from build123d import *

# Parameters (mm, degrees)
EXTRUDE_1_DEPTH = 1.5
FILLET_4_R      = 10
FILLET_7_R      = 1.5
FILLET_8_R      = 3
CHAMFER_1_SIZE  = 0.1
FILLET_9_R      = 2
FILLET_10_R     = 0.5


with BuildPart() as part:
    # 草图1 → 凸台-拉伸1 (new, symmetric)
    with BuildSketch(Plane.XY):
        with BuildLine():
            Line((-130, 3.05), (-130, 14.015709242))
            ThreePointArc((-130, 14.015709242), (-134.003306479, 13.533897344), (-138, 13))
            ThreePointArc((-138, 13), (-144, 12.000000001), (-150, 13))
            Line((-150, 13), (-156.350852961, 24))
            Line((-156.350852961, 24), (-182, 24))
            Line((-182, 24), (-187.773502692, 14))
            Line((-187.773502692, 14), (-189.773502692, 14))
            Line((-189.773502692, 14), (-192.082903768, 18))
            Line((-192.082903768, 18), (-213.75055535, 18))
            Line((-213.75055535, 18), (-220, 7.175644347))
            Line((-220, 7.175644347), (-220, 5.05))
            Line((-220, 5.05), (-215.5, 5.05))
            Line((-215.5, 5.05), (-215.5, 8.3))
            Line((-215.5, 8.3), (-213, 8.3))
            Line((-213, 8.3), (-210.575128869, 12.5))
            Line((-210.575128869, 12.5), (-195.258330249, 12.5))
            Line((-195.258330249, 12.5), (-192.948929172, 8.5))
            Line((-192.948929172, 8.5), (-186.581793069, 8.5))
            Line((-186.581793069, 8.5), (-184.58993464, 5.05))
            Line((-184.58993464, 5.05), (-174.637306696, 5.05))
            Line((-174.637306696, 5.05), (-177.812733177, 10.55))
            Line((-177.812733177, 10.55), (-181.41450816, 10.55))
            Line((-181.41450816, 10.55), (-182.41450816, 12.282050807))
            Line((-182.41450816, 12.282050807), (-178.824573519, 18.5))
            Line((-178.824573519, 18.5), (-159.526279442, 18.5))
            Line((-159.526279442, 18.5), (-153.637306696, 8.3))
            Line((-153.637306696, 8.3), (-150.937306696, 8.3))
            Line((-150.937306696, 8.3), (-150.937306696, 3.05))
            Line((-150.937306696, 3.05), (-150.937306696, -3.05))
            Line((-150.937306696, -3.05), (-150.937306696, -8.3))
            Line((-150.937306696, -8.3), (-153.637306696, -8.3))
            Line((-153.637306696, -8.3), (-159.526279442, -18.5))
            Line((-159.526279442, -18.5), (-178.824573519, -18.5))
            Line((-178.824573519, -18.5), (-182.41450816, -12.282050807))
            Line((-182.41450816, -12.282050807), (-181.41450816, -10.55))
            Line((-181.41450816, -10.55), (-177.812733177, -10.55))
            Line((-177.812733177, -10.55), (-174.637306696, -5.05))
            Line((-174.637306696, -5.05), (-184.58993464, -5.05))
            Line((-184.58993464, -5.05), (-186.581793069, -8.5))
            Line((-186.581793069, -8.5), (-192.948929172, -8.5))
            Line((-192.948929172, -8.5), (-195.258330249, -12.5))
            Line((-195.258330249, -12.5), (-210.575128869, -12.5))
            Line((-210.575128869, -12.5), (-213, -8.3))
            Line((-213, -8.3), (-215.5, -8.3))
            Line((-215.5, -8.3), (-215.5, -5.05))
            Line((-215.5, -5.05), (-220, -5.05))
            Line((-220, -5.05), (-220, -7.175644347))
            Line((-220, -7.175644347), (-213.75055535, -18))
            Line((-213.75055535, -18), (-192.082903768, -18))
            Line((-192.082903768, -18), (-189.773502692, -14))
            Line((-189.773502692, -14), (-187.773502692, -14))
            Line((-187.773502692, -14), (-182, -24))
            Line((-182, -24), (-156.350852961, -24))
            Line((-156.350852961, -24), (-150, -13))
            ThreePointArc((-150, -13), (-144, -12), (-138, -13))
            ThreePointArc((-138, -13), (-134.003306479, -13.533897343), (-130, -14.015709241))
            Line((-130, -14.015709242), (-130, -3.05))
            Line((-130, -3.05), (-145.937306696, -3.05))
            Line((-145.937306696, -3.05), (-145.937306696, 3.05))
            Line((-145.937306696, 3.05), (-130, 3.05))
        make_face()
    extrude(amount=EXTRUDE_1_DEPTH, both=True)

    # 圆角4
    fillet_4_edges = [part.edges().sort_by_distance(p)[0] for p in [
        (-138, 13, 0),
        (-138, -13, 0),
        (-150, -13, 0),
        (-150, 13, 0),
    ]]
    fillet(fillet_4_edges, radius=FILLET_4_R)

    # 圆角7
    fillet_7_edges = [part.edges().sort_by_distance(p)[0] for p in [
        (-187.773502692, -14, 0),
        (-189.773502692, -14, 0),
        (-210.575128869, -12.5, 0),
        (-195.258330249, -12.5, 0),
        (-186.581793069, -8.5, 0),
        (-181.41450816, -10.55, 0),
        (-182.41450816, -12.282050807, 0),
        (-178.824573519, -18.5, 0),
        (-159.526279442, -18.5, 0),
        (-159.526279442, 18.5, 0),
        (-178.824573519, 18.5, 0),
        (-182.41450816, 12.282050807, 0),
        (-181.41450816, 10.55, 0),
        (-186.581793069, 8.5, 0),
        (-195.258330249, 12.5, 0),
        (-210.575128869, 12.5, 0),
        (-189.773502692, 14, 0),
        (-187.773502692, 14, 0),
    ]]
    fillet(fillet_7_edges, radius=FILLET_7_R)

    # 圆角8
    fillet_8_edges = [part.edges().sort_by_distance(p)[0] for p in [
        (-156.350852961, -24, 0),
        (-182, -24, 0),
        (-192.082903768, -18, 0),
        (-213.75055535, -18, 0),
        (-192.948929172, -8.5, 0),
        (-184.58993464, -5.05, 0),
        (-177.812733177, -10.55, 0),
        (-177.812733177, 10.55, 0),
        (-184.58993464, 5.05, 0),
        (-192.948929172, 8.5, 0),
        (-213.75055535, 18, 0),
        (-192.082903768, 18, 0),
        (-182, 24, 0),
        (-156.350852961, 24, 0),
    ]]
    fillet(fillet_8_edges, radius=FILLET_8_R)

    # 倒角1
    chamfer_1_edges = [part.edges().sort_by_distance(p)[0] for p in [
        (-145.937306696, 3.05, 0),
        (-145.937306696, -3.05, 0),
        (-220, -5.05, 0),
        (-215.5, -5.05, 0),
        (-215.5, 5.05, 0),
        (-220, 5.05, 0),
    ]]
    chamfer(chamfer_1_edges, length=CHAMFER_1_SIZE)

    # 圆角9
    fillet_9_edges = [part.edges().sort_by_distance(p)[0] for p in [
        (-130, 14.015709242, 0),
        (-130, -14.015709241, 0),
    ]]
    fillet(fillet_9_edges, radius=FILLET_9_R)

    # 圆角10
    fillet_10_edges = [part.edges().sort_by_distance(p)[0] for p in [
        (-174.637306696, -5.05, 0),
        (-174.637306696, 5.05, 0),
    ]]
    fillet(fillet_10_edges, radius=FILLET_10_R)


solid = part.part
Here's how the part is built. I have some questions about the finished solid (model axes, mm). A direction names the side the tool comes from. Give positions to 0.01 mm unless a question says otherwise; leave off trailing zeros. Order: outer loops, then holes, each group sorted by start corner. A loop starts at its lowest first (then second) coordinate and runs counter-clockwise, first axis right, second up. Notation, with made-up numbers: (62, -29) -> (97, -29) arc R17 ccw to (97, -19) -> close; hole circle Ø11 at (-38.75, -31). An arc over 180 degrees is marked (long way). One line per item, written item: value. Start each with the question number.
1. Imagine slicing it at B-B, the plane x = -184.5. List the corners of the cut face in (y, z) for me, plus the area to 3 significant figures.
2. For faces 4 (the face through (-134.65, 13.45, 0.02)), 5 (the face through (-192.736, 8.913, 0.021)), 6 (the face through (-179, 5.05, 0)), which set-ups out of +Z, -Z, +X, -X, +Y, -Y let a thin tool reach every point of the face, with its end or its side?
3. We'd pull the mould along Y, two halves only. Please class faces 1 (the face through (-179, -7, 1.5)), 2 (the face through (-148, -13, 0)), 3 (the face through (-184.377, 5.463, 0.021)): released by +Y, released by -Y, zero draft, split by the parting line, or undercut.
4. Imagine slicing it at C-C, the plane y = -4. List the corners of the cut face in (x, z) for me.
5. Imagine slicing it at D-D, the plane x = -150. List the corners of the cut face in (y, z) for me.
6. Imagine slicing it at A-A, the plane x = -169.5. List the corners of the cut face in (y, z) for me.
7. Will these pins go through, and if not, where does the flat tip stop? pin 1 Ø1.5 at (x, z) = (-137, 0) entering from +Y; pin 2 Ø1.5 at (x, z) = (-218, 0) entering from -Y; pin 3 Ø1.2 at (x, z) = (-214, 0) entering from +Y.
8. I need wall thicknesses on probe 1 along Y at (x, z) = (-200, 0.2); probe 2 along X at (y, z) = (-6.5, 0.1); probe 3 along Y at (x, z) = (-163.5, -0.15). Which ranges of each line are inside material? Lowest first, please. Write a range as from..to.
Values follow:
1. outline: (-19.67, -1.5) -> (-5.54, -1.5) -> (-5.54, 1.5) -> (-19.67, 1.5) -> close; (5.54, -1.5) -> (19.67, -1.5) -> (19.67, 1.5) -> (5.54, 1.5) -> close
1. area: 84.8 mm2
2. face 4: +Z, -Z, +Y
2. face 5: +Z, -Z
2. face 6: +Z, -Z, -X
3. face 1: zero draft
3. face 2: released by -Y
3. face 3: undercut
4. outline: (-150.94, -1.5) -> (-130, -1.5) -> (-130, 1.5) -> (-150.94, 1.5) -> close
5. outline: (-14.28, -1.5) -> (14.28, -1.5) -> (14.28, 1.5) -> (-14.28, 1.5) -> close
6. outline: (-24, -1.5) -> (-18.5, -1.5) -> (-18.5, 1.5) -> (-24, 1.5) -> close; (18.5, -1.5) -> (24, -1.5) -> (24, 1.5) -> (18.5, 1.5) -> close
7. pin 1: stops at y = 13.24
7. pin 2: stops at y = -11.94
7. pin 3: stops at y = 17.66
8. probe 1: y = -18..-12.5, 12.5..18
8. probe 2: x = -220..-215.5, -185.43..-175.47, -150.94..-130
8. probe 3: y = -24..-18.5, 18.5..24
